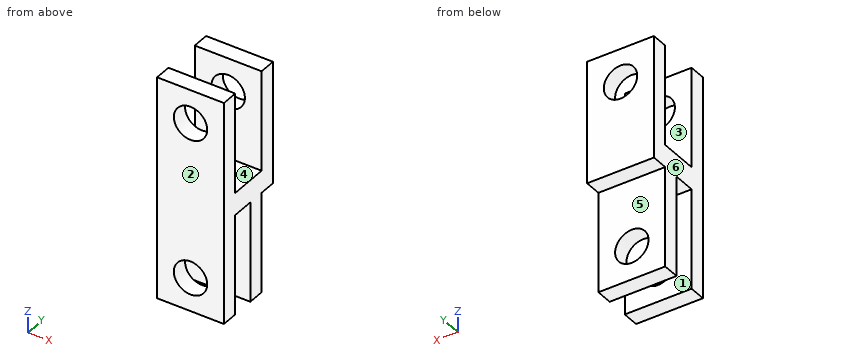
```python
from build123d import *

# Parameters (mm, degrees)
BOSS_EXTRUDE1_DEPTH     = 6
SKETCH2_R               = 1.5
CUT_EXTRUDE1_DEPTH      = 1
CUT_EXTRUDE1_DEPTH_BACK = 7.5


with BuildPart() as part:
    # Sketch1 → Boss-Extrude1 (new body)
    with BuildSketch(Plane(origin=(0, 0, 0), x_dir=(0, 0, -1), z_dir=(1, 0, 0))):
        Polygon((0, 0), (-20, 0), (-20, 1.5), (-11, 1.5), (-11, 5), (-20, 5), (-20, 6.5), (-9, 6.5), (-9, 5), (0, 5), (0, 3.5), (-9, 3.5), (-9, 1.5), (0, 1.5), align=None)
    extrude(amount=BOSS_EXTRUDE1_DEPTH)

    # Sketch2 → Cut-Extrude1 (cut, two sides)
    with BuildSketch(Plane.XZ) as cut_extrude1_sk:
        with Locations((3, 3)):
            Circle(SKETCH2_R)
        with Locations((3, 17)):
            Circle(SKETCH2_R)
    extrude(amount=CUT_EXTRUDE1_DEPTH, mode=Mode.SUBTRACT)
    extrude(cut_extrude1_sk.sketch, amount=-CUT_EXTRUDE1_DEPTH_BACK, mode=Mode.SUBTRACT)


solid = part.part
```
Read the model definition and answer for the solid it produces. Units are mm, in the model's axes. Face numbers are marked on the shaded views. A direction names the side the tool comes from. Give positions to 0.01 mm unless a question says otherwise; leave off trailing zeros. Loops run counter-clockwise (first coordinate to the right, second up) from the corner with the lowest first, then second, coordinate; pieces in that order, holes last.
Item 1: Each of these flat-tipped pins is pushed along its axis until it touches: pin 1 Ø1.8 at (x, z) = (4.5, 6) entering from +Y; pin 2 Ø1.8 at (x, y) = (2, 4) entering from +Z. Where does it stop, or does it pass through?
Item 2: Find the intervals of material crossed by line 1 along Z through (x, y) = (3, 0.6); line 2 along Y through (x, z) = (1.45, 5.75); line 3 along Z through (x, y) = (3, 4.55), in increasing order.
Item 3: The part is cut by section C-C (z = 12). Write down the section's boundary in (x, y), and give its area (3 significant figures).
Item 4: The part is cut by section A-A (x = 3). Give the number of separate pieces and of enclosed holes in the cut face, and give its area (3 significant figures).
Item 5: The part is cut by section D-D (y = 5.5). Write down the section's boundary in (x, z).
Item 6: The part is cut by section B-B (z = 3). Write down the section's boundary in (x, y).
Item 7: The mould has two halves that part along Y. Classify the marked faces 4, 5 and 6: released by +Y, released by -Y, zero draft, split by the parting line, or undercut.
Item 8: For the marked faces 1, 2 and 3, determine the directions among +Z, -Z, +X, -X, +Y, -Y from which every point of the face is accessible in a straight line to the end or side of a thin tool.
Taken from the geometry:
1. pin 1: stops at y = 5
1. pin 2: stops at z = 11
2. line 1: z = 0 to 1.5, 4.5 to 15.5, 18.5 to 20
2. line 2: y = 0 to 1.5, 3.5 to 5
2. line 3: z = 0 to 1.5, 4.5 to 11
3. outline: (0, 0) - (6, 0) - (6, 1.5) - (0, 1.5) - close; (0, 5) - (6, 5) - (6, 6.5) - (0, 6.5) - close
3. area: 18.0 mm2
4. separate pieces: 5
4. enclosed holes: 0
4. area: 49.0 mm2
5. outline: (0, 9) - (6, 9) - (6, 20) - (0, 20) - close; hole circle Ø3 at (3, 17)
6. outline: (0, 0) - (1.5, 0) - (1.5, 1.5) - (0, 1.5) - close; (0, 3.5) - (1.5, 3.5) - (1.5, 5) - (0, 5) - close; (4.5, 0) - (6, 0) - (6, 1.5) - (4.5, 1.5) - close; (4.5, 3.5) - (6, 3.5) - (6, 5) - (4.5, 5) - close
7. face 4: undercut
7. face 5: released by +Y
7. face 6: zero draft
8. face 1: -Z, +X, -X
8. face 2: +Z, -Z, +X, -X, -Y
8. face 3: +Z, +X, -X
